Autodesk Inventor part; units mm, degrees
ref_plane "YZ Plane" through (0, 0, 0) normal (1, 0, 0) x (0, 1, 0)
ref_plane "XZ Plane" through (0, 0, 0) normal (0, 1, 0) x (-1, 0, 0)
ref_plane "XY Plane" through (0, 0, 0) normal (0, 0, 1) x (1, 0, 0)
sketch "Sketch1" plane through (0, 0, 0) normal (0, 1, 0) x (-1, 0, 0)
  line L0 (0, 0) -> (0, -2.75)
  line L1 (0, 0) -> (9.5, 0)
  line L2 (9.5, 0) -> (9.5, -1.5)
  line L3 (9.5, -1.5) -> (2, -1.5)
  line L4 (2, -1.5) -> (0.75, -2.75)
  line L5 (2, -1.5) -> (3.7678, -1.5) construction
  line L6 (0.75, -2.75) -> (0, -2.75)
  dimension "d0" = 2.75
  dimension "d1" = 9.5
  dimension "d2" = 1.5
  dimension "d3" = 7.5
  dimension "d4" = 135
revolve "Revolution1" add sketch "Sketch1" angle 360 about axis through (0, 0, 0) along (-1, 0, 0)
thread "Thread1"
fillet "Fillet1" radius 0.25 2 edges at (-0.75, 0, 2.75) (0, 0, 2.75)
sketch "Sketch2" plane through (0, 0, 0) normal (1, 0, 0) x (0, 0, -1)
  line L0 (-1.5, 0.5) -> (1.5, 0.5)
  line L1 (1.5, 0.5) -> (1.5, -0.5)
  line L2 (1.5, -0.5) -> (-1.5, -0.5)
  line L3 (-1.5, -0.5) -> (-1.5, 0.5)
  line L4 (-1.5, 0.5) -> (1.5, -0.5) construction
  line L5 (1.5, 0.5) -> (-1.5, -0.5) construction
  line L6 (0.5, 1.5) -> (-0.5, 1.5)
  line L7 (-0.5, 1.5) -> (-0.5, -1.5)
  line L8 (-0.5, -1.5) -> (0.5, -1.5)
  line L9 (0.5, -1.5) -> (0.5, 1.5)
  line L10 (0.5, 1.5) -> (-0.5, -1.5) construction
  line L11 (-0.5, 1.5) -> (0.5, -1.5) construction
  point P0 (0, 0)
  point P1 (0.5, 0.5)
  point P2 (-0.5, 0.5)
  point P3 (-0.5, -0.5)
  point P4 (0.5, -0.5)
  dimension "d9" = 3
  dimension "d10" = 1
  dimension "d11" = 1
  dimension "d12" = 3
extrude "Extrusion1" cut sketch "Sketch2" against normal blind 1.5
chamfer "Chamfer1" distance 0.25 angle 45 1 edges at (-9.5, 0, 1.5)
properties part number "M3_Short_Bolt" material "Steel, Alloy"
Can you work these out from the model? Positions are in its coordinate system, mm. A direction names the side the tool comes from. Round coordinates to 2 decimals unless told otherwise and drop trailing zeros. Loops run counter-clockwise (first coordinate to the right, second up) from the corner with the lowest first, then second, coordinate; pieces in that order, holes last. Notation, with made-up numbers: (42, -9.75) - (87, -9.75) arc R13 ccw to (87, 1.25) - close; hole circle Ø1 at (72, -16.5). An arc over 180 degrees is marked (long way). Answer in a Markdown table with one row per item. Add a question column.
Q1. We'd pull the mould along Y, two halves only. Please class faces 4 (the flat face through (-9.5, 0, 0)), 5 (the flat face through (-1, -0.5, -1)), 6 (the cylindrical face through (-0.445, 2.727, 0.358)): pulls with the +Y half, pulls with the -Y half, needs draft (parallel to the pull), parting line crosses it, or undercut.
Q2. For pin 1 Ø0.8 at (x, y) = (-0.5, 1) entering from +Z; pin 2 Ø1 at (y, z) = (1.5, -1) entering from -X; pin 3 Ø0.5 at (x, y) = (-0.5, 1) entering from -Z, each with a flat end and sliding along its axis, tell me the tip position at first contact or that it passes through.
Q3. I need wall thicknesses on L1, parallel to Y at x = -4, z = 0; L2, parallel to X at y = 0, z = -0.2; L3, parallel to Y at x = -5, z = -1.3. Which ranges of each line are inside material? Lowest first, please.
Q4. I want a section at A-A on x = -5. List the corners of the cut face in (y, z) for me, and give its area (3 significant figures).
Q5. Which directions (+Z, -Z, +X, -X, +Y, -Y) give clear straight access to the entire face, cutting with the end or side of a thin tool? Please do faces 1 (the cylindrical face through (-5.57, 0.07, 1.5)), 2 (the flat face through (0, 1, -1)), 3 (the flat face through (-1, -0.5, 1)).
A:
| question | item | result |
|---|---|---|
| 1 | face 4 | needs draft |
| 1 | face 5 | undercut |
| 1 | face 6 | parting line crosses it |
| 2 | pin 1 | z = 2.68 |
| 2 | pin 2 | x = -9.45 |
| 2 | pin 3 | z = -2.65 |
| 3 | L1 | -1.5 to 1.5 |
| 3 | L2 | -9.5 to -1.5 |
| 3 | L3 | -0.75 to 0.75 |
| 4 | outline | circle Ø3 at (0, 0) |
| 4 | area | 7.07 mm^2 |
| 5 | face 1 | -X |
| 5 | face 2 | +Z, -Z, +X, +Y, -Y |
| 5 | face 3 | +X |
